```python
from build123d import *

# Parameters (mm, degrees)
BOSS_EXTRUDE1_DEPTH = 2
BOSS_EXTRUDE3_DEPTH = 20
SKETCH7_R           = 4.5
CUT_EXTRUDE1_DEPTH  = 0.2
SKETCH8_R           = 3
CUT_EXTRUDE2_DEPTH  = 38.831864876
FILLET3_R           = 2
FILLET4_R           = 1
FILLET5_R           = 0.8


with BuildPart() as part:
    # Sketch1 → Boss-Extrude1 (new body)
    with BuildSketch(Plane.XY):
        Polygon((-2.5, 30), (22.5, 30), (22.5, -3.215927905), (-3.5, -23.03885463), (-3.5, -30), (-22.5, -30), (-22.5, -16.5), (-2.5, 0), align=None)
    extrude(amount=-BOSS_EXTRUDE1_DEPTH)

    # Sketch6 → Boss-Extrude3 (add)
    with BuildSketch(Plane(origin=(0, 25, 0), x_dir=(-1, 0, 0), z_dir=(0, 1, 0))):
        Polygon((2.5, 0), (-12, 5), (-19, 0), align=None)
    extrude(amount=-BOSS_EXTRUDE3_DEPTH)

    # Sketch7 → Cut-Extrude1 (cut)
    with BuildSketch(Plane(origin=(-0.265674814, 0, 0.770456961), x_dir=(0.9453729816262723, 0, 0.3259906833194039), z_dir=(-0.3259906833194039, 0, 0.9453729816262723))):
        with Locations((5.305498371, 15)):
            Circle(SKETCH7_R)
    extrude(amount=-CUT_EXTRUDE1_DEPTH, mode=Mode.SUBTRACT)

    # Sketch8 → Cut-Extrude2 (cut, through all)
    with BuildSketch(Plane.XY):
        with Locations((1.279211248, -0.215927905)):
            Circle(SKETCH8_R)
    extrude(amount=-CUT_EXTRUDE2_DEPTH, mode=Mode.SUBTRACT)

    # Fillet3
    fillet3_edges = [part.edges().sort_by_distance(p)[0] for p in [
        (12, 15, 5),
    ]]
    fillet(fillet3_edges, radius=FILLET3_R)

    # Fillet4
    fillet4_edges = [part.edges().sort_by_distance(p)[0] for p in [
        (11.964055432, 5, 4.752278398),
        (15.919669033, 5, 2.200236405),
        (4.262440156, 5, 2.331875916),
        (4.262440156, 25, 2.331875916),
        (11.964055432, 25, 4.752278398),
        (15.919669033, 25, 2.200236405),
    ]]
    fillet(fillet4_edges, radius=FILLET4_R)

    # Fillet5
    fillet5_edges = [part.edges().sort_by_distance(p)[0] for p in [
        (-2.5, 0, -1),
        (-22.5, -16.5, -1),
        (-3.5, -23.03885463, -1),
        (22.5, -3.215927905, -1),
        (-2.5, 30, -1),
        (22.5, 30, -1),
    ]]
    fillet(fillet5_edges, radius=FILLET5_R)


solid = part.part
```
Geometry: final body of the model. Coordinates: model frame, mm. A direction names the side the tool comes from. Round coordinates to 2 decimals unless told otherwise and drop trailing zeros. Order: outer loops, then holes, each group sorted by start corner. A loop starts at its lowest first (then second) coordinate and runs counter-clockwise, first axis right, second up. Notation, with made-up numbers: (74, 75) - (89, 75) arc R13 cw to (89, 96) - close; hole circle Ø10 at (-12.5, -10.75). An arc over 180 degrees is marked (long way). Use CSV: the item, a comma, the result in double quotes. Start each with the question number.
Q1. Mould query, pull axis Y, two halves, no side actions, for faces 1 (the face through (4.45, 24.699, 2.095)), 2 (the face through (-3.5, -27, -1)), 3 (the face through (9, 5, 1)), 4 (the face through (-1.101, -2.041, -0.986)). Classes: +Y half, -Y half, draft (parallel to the pull), parting line (faces both ways), or undercut.
Q2. Section query A-A (y = 7.5). Return loops of the section in (x, z), and give its area (3 significant figures).
Q3. Section query C-C (x = -4.5). Return loops of the section in (y, z), and give its area (3 significant figures).
Q4. Section query D-D (y = 17). Return loops of the section in (x, z).
Q5. Section query B-B (y = -2). Return loops of the section in (x, z).
Q6. Access query for faces 5 (the face through (4.45, 5.301, 2.095)), 6 (the face through (-2.5, 15, -1)). Directions: +Z, -Z, +X, -X, +Y, -Y. A direction counts if a zero-diameter tool reaches every point of the face in a straight line with its end or side. Return the directions, or none.
Q7. Material intervals for line 1 along Z through (x, y) = (-19, -22.5); line 2 along X through (y, z) = (15, -0.25); line 3 along Y through (x, z) = (8.5, 2.75), sorted ascending. Write a range as from..to.
Q8. First-contact query: pin 1 (4 mm diameter, centred on x = -14.5, z = 3.5, fed in from +Y); pin 2 (12 mm diameter, centred on x = -15, y = -14, fed in from +Z); pin 3 (3 mm diameter, centred on y = 4.5, z = -0.5, fed in from -X); pin 4 (1 mm diameter, centred on x = 7, y = 19.5, fed in from +Z). Flat tips, straight axial feed; report the tip coordinate or a pass-through.
Result set:
1,face 1,"+Y half"
1,face 2,"draft"
1,face 3,"-Y half"
1,face 4,"undercut"
2,outline,"(-2.5, -2) - (22.5, -2) - (22.5, 0) - (19, 0) - (12.84, 4.4) arc R2 ccw to (11.02, 4.66) - (-2.5, 0) - close"
2,area,"104 mm2"
3,outline,"(-30, -2) - (-1.65, -2) - (-1.65, 0) - (-30, 0) - close"
3,area,"56.7 mm2"
4,outline,"(-2.5, -2) - (22.5, -2) - (22.5, 0) - (19, 0) - (12.84, 4.4) arc R2 ccw to (11.02, 4.66) - (8.56, 3.81) - (8.63, 3.63) - (1, 1) - (0.94, 1.19) - (-2.5, 0) - close"
5,outline,"(-4.92, -2) - (-1.13, -2) - (-1.13, 0) - (-4.92, 0) - close; (3.69, -2) - (22.5, -2) - (22.5, 0) - (3.69, 0) - close"
6,face 5,"+Z, -X, -Y"
6,face 6,"+Z, -Z, -X, +Y"
7,line 1,"z = -2..0"
7,line 2,"x = -2.5..22.5"
7,line 3,"y = 5..25"
8,pin 1,"passes through"
8,pin 2,"stops at z = 0"
8,pin 3,"stops at x = -2.5"
8,pin 4,"stops at z = 3.45"
